from build123d import *

# Parameters (mm, degrees)
F0_R            = 2.15265
F0_R_2          = 3.96875
F0_W            = 9.525
F0_H            = 3.175
F1_DEPTH        = 9.525
F2_R            = 2.15265
F3_REACH        = 43.3958636501
F5_R            = 3.96875
F6_DEPTH        = 3.175
F8_DEPTH        = 9.525
F8_COPIES_COUNT = 3
F8_COPIES_ANGLE = 180
F9_R            = 0.762


# Not quite as in the source:
# - a feature of the source that left no trace in its solid (it failed there, or was rolled back) is left out
# - a pattern or mirror of a feature is missing from the dataset's text; its kind, count and spacing are read off the source's solid


with BuildPart() as f1:
    # F0 (on Top) → F1 (new body)
    with BuildSketch(Plane.XY):
        with BuildLine():
            Line((3.96875, 15.08125), (-3.96875, 15.08125))
            Line((-3.96875, 15.08125), (-3.96875, 21.8677764859))
            ThreePointArc((-3.96875, 21.8677764859), (0, -22.225), (3.96875, 21.8677764859))
            Line((3.96875, 21.8677764859), (3.96875, 15.08125))
        make_face()
        with Locations((-11.7865861589, -11.7865861589)):
            Circle(F0_R, mode=Mode.SUBTRACT)
        with Locations((11.7865861589, -11.7865861589)):
            Circle(F0_R, mode=Mode.SUBTRACT)
        with Locations((-11.7865861589, 11.7865861589)):
            Circle(F0_R, mode=Mode.SUBTRACT)
        Circle(F0_R_2, mode=Mode.SUBTRACT)
        with Locations((0, 8.73125)):
            Rectangle(F0_W, F0_H, mode=Mode.SUBTRACT)
        with Locations((11.7865861589, 11.7865861589)):
            Circle(F0_R, mode=Mode.SUBTRACT)
    extrude(amount=F1_DEPTH)

    f3_end = f1.faces().sort_by_distance((-3.96875, 0, 4.7625))[0]
    # F2 (on face) → F3 (cut, up to a face of the model that its end follows)
    with BuildSketch(Plane(origin=(0, 15.08125, 0), x_dir=(-1, 0, 0), z_dir=(0, 1, 0))):
        with Locations((0, 4.7625)):
            Circle(F2_R)
    f3_long = extrude(amount=-F3_REACH, mode=Mode.PRIVATE)
    add(split(f3_long, bisect_by=f3_end, keep=Keep.ALL, mode=Mode.PRIVATE).solids().sort_by_distance((0, 15.08125, 4.7625))[0], mode=Mode.SUBTRACT)

    # F5 (on face) → F6 (cut, through all)
    with BuildSketch(Plane(origin=(0, 0, 0), x_dir=(1, 0, 0), z_dir=(0, 0, -1))):
        with Locations((11.7865861589, -11.7865861589)):
            Circle(F5_R)
        with Locations((-11.7865861589, 11.7865861589)):
            Circle(F5_R)
    extrude(amount=-F6_DEPTH, mode=Mode.SUBTRACT)

    # F7 (on face) → F8 (cut, through all)
    with BuildSketch(Plane(origin=(0, 0, 0), x_dir=(1, 0, 0), z_dir=(0, 0, -1))):
        with BuildLine():
            ThreePointArc((-17.3148424047, -11.229543123), (-14.7565267097, -7.0906978311), (-9.9206262673, -6.5530302219))
            Line((-9.9206262673, -6.5530302219), (-7.6236791242, -4.2560830788))
            ThreePointArc((-7.6236791242, -4.2560830788), (-8.73125, 0), (-7.6236791242, 4.2560830788))
            Line((-7.6236791242, 4.2560830788), (-9.9206262673, 6.5530302219))
            ThreePointArc((-9.9206262673, 6.5530302219), (-14.7565267097, 7.0906978311), (-17.3148424047, 11.229543123))
            ThreePointArc((-17.3148424047, 11.229543123), (-20.6375, 0), (-17.3148424047, -11.229543123))
        make_face()
    f8 = extrude(amount=-F8_DEPTH, mode=Mode.SUBTRACT)

    # F8_copies: F8 ×3 about axis
    f8_copies_axis = Axis((0, 0, 0), (0, 0, 1))
    for i in range(1, F8_COPIES_COUNT):
        add(f8.rotate(f8_copies_axis, i * F8_COPIES_ANGLE / (F8_COPIES_COUNT - 1)), mode=Mode.SUBTRACT)

    # F9
    f9_edges = [f1.edges().sort_by_distance(p)[0] for p in [
        (-17.314842, -11.229543, 4.7625),
        (-9.920626, -6.55303, 4.7625),
        (-7.623679, -4.256083, 4.7625),
        (-7.623679, 4.256083, 4.7625),
        (-9.920626, 6.55303, 4.7625),
        (-17.314842, 11.229543, 4.7625),
        (3.96875, 21.867776, 4.7625),
        (-3.96875, 21.867776, 4.7625),
        (11.229543, -17.314842, 4.7625),
        (-11.229543, -17.314842, 4.7625),
        (6.55303, -9.920626, 4.7625),
        (-6.55303, -9.920626, 4.7625),
        (4.256083, -7.623679, 4.7625),
        (-4.256083, -7.623679, 4.7625),
        (17.314842, 11.229543, 4.7625),
        (17.314842, -11.229543, 4.7625),
        (9.920626, 6.55303, 4.7625),
        (7.623679, 4.256083, 4.7625),
        (7.623679, -4.256083, 4.7625),
        (9.920626, -6.55303, 4.7625),
    ]]
    fillet(f9_edges, radius=F9_R)


solid = f1.part
Input: part model. Units: mm. Frame: model coordinates. A direction names the side the tool comes from. Give positions to 0.01 mm unless a question says otherwise; leave off trailing zeros. Order: outer loops, then holes, each group sorted by start corner. A loop starts at its lowest first (then second) coordinate and runs counter-clockwise, first axis right, second up. Notation, with made-up numbers: (-37.5, 70) - (12.5, 70) arc R10 ccw to (12.5, 82) - close; hole circle Ø7 at (-22.5, 74.5). An arc over 180 degrees is marked (long way). Answer as a JSON object with one key per item and string values. Group by question number.
Q1. First-contact query: pin 1 Ø2.5 at (x, y) = (-10, -13) entering from -Z (3 decimals); pin 2 Ø4 at (x, z) = (0, 3) entering from +Y; pin 3 Ø3 at (y, z) = (-12, 6) entering from -X; pin 4 Ø3.5 at (x, y) = (11.79, -11.79) entering from +Z. Flat tips, straight axial feed; report the tip coordinate or a pass-through.
Q2. Cut plane A-A, the plane y = 0. Output: boundary loops of the cut face in (x, z) (1 decimal), then the cut area to 3 significant figures.
Q3. Mould query, pull axis X, two halves, no side actions, for faces 4 (the face through (0, 5, 9.525)), 5 (the face through (-10, -10, 3.175)). Classes: pulls with the +X half, pulls with the -X half, needs draft (parallel to the pull), parting line crosses it, or undercut.
Q4. Cut plane B-B, the plane x = 0. Output: boundary loops of the cut face in (y, z) (1 decimal).
Q5. Set-up query: faces 1 (the face through (-0.8, 15.081, 2.6)), 2 (the face through (-8.82, 5.45, 4.7)), 3 (the face through (-2.053, 5.266, 5.409)). Return all of +Z, -Z, +X, -X, +Y, -Y with unobstructed straight access to the full face (end or side cutting, diameter ignored); none if empty.
Q6. Cut plane D-D, the plane y = 18. Output: boundary loops of the cut face in (x, z) (3 decimals), then the cut area to 3 significant figures.
Q7. Cut plane C-C, the plane x = 15. Output: boundary loops of the cut face in (y, z) (3 decimals), then the cut area to 3 significant figures.
Q8. Line query: probe 1 along Y at (x, z) = (15, 2.5); probe 2 along Y at (x, z) = (-9, 1.5); probe 3 along X at (y, z) = (-1, 2). Output: solid intervals per line, ascending.
Results:
{
 "1": {"pin 1": "z = 3.175", "pin 2": "y = 15.08", "pin 3": "x = -19.59", "pin 4": "through"},
 "2": {"outline": "(-22.2, 0) - (-20.6, 0) - (-20.6, 9.5) - (-22.2, 9.5) - close; (-8.7, 0) - (-4, 0) - (-4, 9.5) - (-8.7, 9.5) - close; (4, 0) - (8.7, 0) - (8.7, 9.5) - (4, 9.5) - close; (20.6, 0) - (22.2, 0) - (22.2, 9.5) - (20.6, 9.5) - close", "area": "121 mm^2"},
 "3": {"face 4": "needs draft", "face 5": "undercut"},
 "4": {"outline": "(-22.2, 0) - (-20.6, 0) - (-20.6, 9.5) - (-22.2, 9.5) - close; (-8.7, 0) - (-4, 0) - (-4, 9.5) - (-8.7, 9.5) - close; (4, 0) - (7.1, 0) - (7.1, 2.6) - (4, 2.6) - close; (4, 6.9) - (7.1, 6.9) - (7.1, 9.5) - (4, 9.5) - close; (10.3, 0) - (15.1, 0) - (15.1, 2.6) - (10.3, 2.6) - close; (10.3, 6.9) - (15.1, 6.9) - (15.1, 9.5) - (10.3, 9.5) - close"},
 "5": {"face 1": "+Z, -Z, +Y", "face 2": "+Z, -Z", "face 3": "+Y"},
 "6": {"outline": "(-13.037, 0) - (-3.969, 0) - (-3.969, 9.525) - (-13.037, 9.525) - close; (3.969, 0) - (13.037, 0) - (13.037, 9.525) - (3.969, 9.525) - close", "area": "173 mm^2"},
 "7": {"outline": "(-16.4, 0) - (-7.254, 0) - (-7.254, 9.525) - (-16.4, 9.525) - close; (7.254, 0) - (9.457, 0) - (9.457, 3.175) - (14.116, 3.175) - (14.116, 0) - (16.4, 0) - (16.4, 9.525) - (7.254, 9.525) - close", "area": "159 mm^2"},
 "8": {"probe 1": "-16.4 to -7.25, 7.25 to 9.46, 14.12 to 16.4", "probe 2": "-20.32 to -18.57, -16.59 to -14.61, -8.96 to -5.63, 5.63 to 20.32", "probe 3": "-22.2 to -20.61, -8.67 to -3.84, 3.84 to 8.67, 20.61 to 22.2"}
}
